```python
from build123d import *

# Parameters (mm, degrees)
BASPROSKE_W         = 15
BASPROSKE_H         = 13.2
TOOTHCUT_DEPTH      = 24.947442452
TEETHCUTS_COUNT     = 20
TEETHCUTS_ANGLE     = 342
BORSKE_R            = 4
BORE_DEPTH          = 50.0000508
BOSS_EXTRUDE1_START = -15
BOSS_EXTRUDE1_DEPTH = 15
SKETCH2_R           = 7.2
SKETCH2_R_2         = 6
CUT_EXTRUDE1_DEPTH  = 0.5


with BuildPart() as part:
    # BasProSke → Base-Revolve (revolve)
    with BuildSketch(Plane(origin=(0, 0, 0), x_dir=(1, 0, 0), z_dir=(0, 1, 0)), mode=Mode.PRIVATE) as base_revolve_sk:
        with Locations((7.5, 6.6)):
            Rectangle(BASPROSKE_W, BASPROSKE_H)
    revolve(base_revolve_sk.sketch.rotate(Axis((-10, 0, 0), (1, 0, 0)), 180), axis=Axis((-10, 0, 0), (1, 0, 0)))

    # TooCutSke → ToothCut (cut, through all)
    with BuildSketch(Plane(origin=(0, 0, 0), x_dir=(0, 0, -1), z_dir=(1, 0, 0))):
        with BuildLine():
            ThreePointArc((0.599012827, 10.48189795), (0, 10.499), (-0.599012827, 10.48189795))
            ThreePointArc((-0.599012827, 10.48189795), (-0.986906343, 11.883983562), (-1.777012823, 13.105473306))
            ThreePointArc((-1.777012823, 13.105473306), (0, 13.2254), (1.777012823, 13.105473306))
            ThreePointArc((1.777012823, 13.105473306), (0.986906343, 11.883983562), (0.599012827, 10.48189795))
        make_face()
    toothcut = extrude(amount=TOOTHCUT_DEPTH, mode=Mode.SUBTRACT)

    # TeethCuts: ToothCut ×20 about axis
    teethcuts_axis = Axis((-10, 0, 0), (1, 0, 0))
    for i in range(1, TEETHCUTS_COUNT):
        add(toothcut.rotate(teethcuts_axis, i * TEETHCUTS_ANGLE / (TEETHCUTS_COUNT - 1)), mode=Mode.SUBTRACT)

    # BorSke → Bore (cut, symmetric)
    with BuildSketch(Plane(origin=(0, 0, 0), x_dir=(0, 0, -1), z_dir=(1, 0, 0))):
        with Locations(Location((0, 0, 0), (0, 0, 180))):
            Circle(BORSKE_R)
    extrude(amount=BORE_DEPTH, both=True, mode=Mode.SUBTRACT)

    # Sketch1 → Boss-Extrude1 (add)
    with BuildSketch(Plane.ZY.offset(BOSS_EXTRUDE1_START)):
        with BuildLine():
            Line((-2.856571371, 2.8), (2.856571371, 2.8))
            ThreePointArc((2.856571371, 2.8), (0, 4), (-2.856571371, 2.8))
        make_face()
    extrude(amount=BOSS_EXTRUDE1_DEPTH)

    # Sketch2 → Cut-Extrude1 (cut)
    with BuildSketch(Plane.ZY):
        Circle(SKETCH2_R)
        Circle(SKETCH2_R_2, mode=Mode.SUBTRACT)
    extrude(amount=-CUT_EXTRUDE1_DEPTH, mode=Mode.SUBTRACT)


solid = part.part
```
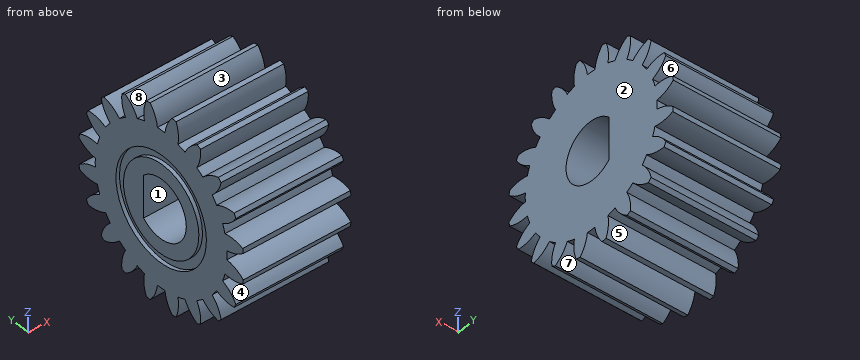
Design review of the part built by this model. Coordinates are the model's own, in mm. Face numbers are marked on the shaded views. A direction names the side the tool comes from. Round coordinates to 2 decimals unless told otherwise and drop trailing zeros. Order: outer loops, then holes, each group sorted by start corner. A loop starts at its lowest first (then second) coordinate and runs counter-clockwise, first axis right, second up. Notation, with made-up numbers: (17.5, 86) - (70.5, 86) arc R28 ccw to (70.5, 110) - close; hole circle Ø1 at (39.25, 19). An arc over 180 degrees is marked (long way). Return JSON: item names as keys, results as strings.
Q1. Consider section B-B on y = 0. Write out the cut boundary in (x, z), plus the area to 3 significant figures.
Computed values:
{"outline": "(0, -10.5) - (15, -10.5) - (15, -4) - (0, -4) - (0, -6) - (0.5, -6) - (0.5, -7.2) - (0, -7.2) - close; (0, 4) - (15, 4) - (15, 10.5) - (0, 10.5) - (0, 7.2) - (0.5, 7.2) - (0.5, 6) - (0, 6) - close", "area": "194 mm2"}
Q2. For pin 1 Ø5 at (y, z) = (0, 0) entering from -X; pin 2 Ø1 at (x, z) = (3.5, 0) entering from -Y; pin 3 Ø1 at (x, z) = (7.5, -9) entering from +Y, all flat-tipped, find the tip position at first contact; note any pin that passes through.
Computed values:
{"pin 1": "passes through", "pin 2": "stops at y = -10.5", "pin 3": "stops at y = 9.55"}
Q3. Wall thickness on L1, parallel to Z at x = 2, y = 8.5; L2, parallel to Y at x = 7.5, z = -9.25; L3, parallel to Z at x = 4, y = -11: over which ranges is each line inside the solid? List them lowest first. Write a range as [from, to].
Computed values:
{"L1": "z = [-9.37, -7.03], [-6.16, 6.16], [7.03, 9.37]", "L2": "y = [-9.42, -8.21], [-5.88, 5.88], [8.21, 9.42]", "L3": "z = [-6.29, -4.61], [-2.76, -0.69], [0.69, 2.76], [4.61, 6.29]"}
Q4. Consider section A-A on z = 0. Write out the cut boundary in (x, y), plus the area to 3 significant figures.
Computed values:
{"outline": "(0, -10.5) - (15, -10.5) - (15, -4) - (0, -4) - (0, -6) - (0.5, -6) - (0.5, -7.2) - (0, -7.2) - close; (0, 2.8) - (15, 2.8) - (15, 10.5) - (0, 10.5) - (0, 7.2) - (0.5, 7.2) - (0.5, 6) - (0, 6) - close", "area": "212 mm2"}
Q5. The part is to be moulded in two halves that separate along Z. For the marked faces 1, 2 and 3, say which applies: pulls with the +Z half, pulls with the -Z half, needs draft (parallel to the pull), parting line crosses it, or undercut.
Computed values:
{"face 1": "undercut", "face 2": "needs draft", "face 3": "pulls with the +Z half"}
Q6. Machinability: for the marked faces 4, 5, 6, 7 and 8, which of the approach directions +Z, -Z, +X, -X, +Y, -Y give a long, thin tool a straight path to every point of the face, cutting with its end or side? Answer none if there is none.
Computed values:
{"face 4": "+X, -X, -Y", "face 5": "+X, -X", "face 6": "+X, -X, +Y", "face 7": "-Z, +X, -X", "face 8": "+Z, +X, -X"}
Q7. Consider section C-C on z = -8.5. Write out the cut boundary in (x, y).
Computed values:
{"outline": "(0, -9.37) - (15, -9.37) - (15, -7.03) - (0, -7.03) - close; (0, -6.16) - (15, -6.16) - (15, 6.16) - (0, 6.16) - close; (0, 7.03) - (15, 7.03) - (15, 9.37) - (0, 9.37) - close"}
